Can you work these out from the model? Positions are in its coordinate system, mm. Face numbers are marked on the shaded views. Give positions to 0.01 mm unless a question says otherwise; leave off trailing zeros. Order: outer loops, then holes, each group sorted by start corner. A loop starts at its lowest first (then second) coordinate and runs counter-clockwise, first axis right, second up. Notation, with made-up numbers: (19, 57.5) - (34, 57.5) arc R27 ccw to (34, 90.5) - close; hole circle Ø5 at (88.5, 8.25). An arc over 180 degrees is marked (long way). Answer as CSV lines item,"result".
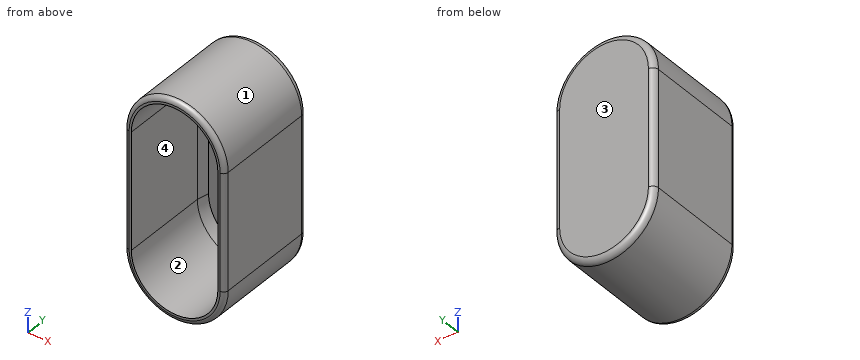
```python
from build123d import *

# Parameters (mm, degrees)
F1_DEPTH  = 15
F5_DEPTH  = 2
F10_DEPTH = 1.5
F11_R     = 1
F12_R     = 0.8


with BuildPart() as f1:
    # F0 (on Front) → F1 (new body)
    with BuildSketch(Plane.XZ):
        with BuildLine():
            Line((8.8, 0), (8.8, 20.5))
            ThreePointArc((8.8, 20.5), (0, 29.3), (-8.8, 20.5))
            Line((-8.8, 20.5), (-8.8, 0))
            ThreePointArc((-8.8, 0), (0, -8.8), (8.8, 0))
        make_face()
        with BuildLine():
            ThreePointArc((-7.6, 20.5), (0, 28.1), (7.6, 20.5))
            Line((7.6, 20.5), (7.6, 0))
            ThreePointArc((7.6, 0), (0, -7.6), (-7.6, 0))
            Line((-7.6, 0), (-7.6, 20.5))
        make_face(mode=Mode.SUBTRACT)
    extrude(amount=F1_DEPTH)

    # F4 (on face) → F5 (join)
    with BuildSketch(Plane(origin=(0, 0, 0), x_dir=(-1, 0, 0), z_dir=(0, 1, 0))):
        with BuildLine():
            ThreePointArc((8.8, 20.5), (0, 29.3), (-8.8, 20.5))
            Line((-8.8, 20.5), (-8.8, 0))
            ThreePointArc((-8.8, 0), (0, -8.8), (8.8, 0))
            Line((8.8, 0), (8.8, 20.5))
        make_face()
    extrude(amount=F5_DEPTH)

    # F3 (on offset) → F8 section 0
    with BuildSketch(Plane(origin=(0, 2.4, 0), x_dir=(-1, 0, 0), z_dir=(0, 1, 0))):
        with BuildLine():
            ThreePointArc((7.1, 20.5), (0, 27.6), (-7.1, 20.5))
            Line((-7.1, 20.5), (-7.1, 0))
            ThreePointArc((-7.1, 0), (0, -7.1), (7.1, 0))
            Line((7.1, 0), (7.1, 20.5))
        make_face()
    # F7 (on offset) → F8 section 1
    with BuildSketch(Plane(origin=(0, 0, 0), x_dir=(-1, 0, 0), z_dir=(0, 1, 0))):
        with BuildLine():
            Line((7.6, 0), (7.6, 20.5))
            ThreePointArc((7.6, 20.5), (0, 28.1), (-7.6, 20.5))
            Line((-7.6, 20.5), (-7.6, 0))
            ThreePointArc((-7.6, 0), (0, -7.6), (7.6, 0))
        make_face()
    loft(mode=Mode.SUBTRACT)

    # F9 (on face) → F10 (join)
    with BuildSketch(Plane(origin=(0, 2, 0), x_dir=(-1, 0, 0), z_dir=(0, 1, 0))):
        with BuildLine():
            ThreePointArc((8.8, 20.5), (0, 29.3), (-8.8, 20.5))
            Line((-8.8, 20.5), (-8.8, 0))
            ThreePointArc((-8.8, 0), (0, -8.8), (8.8, 0))
            Line((8.8, 0), (8.8, 20.5))
        make_face()
    extrude(amount=F10_DEPTH)

    # F11
    f11_edges = [f1.edges().sort_by_distance(p)[0] for p in [
        (0, 3.5, -8.8),
    ]]
    fillet(f11_edges, radius=F11_R)

    # F12
    f12_edges = [f1.edges().sort_by_distance(p)[0] for p in [
        (8.8, -15, 10.25),
    ]]
    fillet(f12_edges, radius=F12_R)


solid = f1.part
```
1) I want a section at D-D on y = 1.5. Write out the boundary of the cut face in (x, z) (1 decimal).
Answer block:
outline,"(-8.8, 0) arc R8.8 ccw to (8.8, 0) - (8.8, 20.5) arc R8.8 ccw to (-8.8, 20.5) - close; hole (-7.3, 0) arc R7.3 ccw to (7.3, 0) - (7.3, 20.5) arc R7.3 ccw to (-7.3, 20.5) - close"
2) I want a section at A-A on y = -10.5. Write out the boundary of the cut face in (x, z).
Answer block:
outline,"(-8.8, 0) arc R8.8 ccw to (8.8, 0) - (8.8, 20.5) arc R8.8 ccw to (-8.8, 20.5) - close; hole (-7.6, 0) arc R7.6 ccw to (7.6, 0) - (7.6, 20.5) arc R7.6 ccw to (-7.6, 20.5) - close"
3) If we mould it in two halves opening along X, with no side actions, what happens to the marked faces 1, 2, 3 and 4? For each: +X half, -X half, draft (parallel to the pull), parting line (faces both ways), or undercut.
Answer block:
face 1,"parting line"
face 2,"undercut"
face 3,"draft"
face 4,"undercut"
4) I need wall thicknesses on line 1 along X through (y, z) = (-2.75, 6); line 2 along Y through (x, z) = (-1.75, 18.5); line 3 along Z through (x, y) = (4, -7). Which ranges of each line are inside material? Lowest first, please. Write a range as [from, to].
Answer block:
line 1,"[-8.8, -7.6], [7.6, 8.8]"
line 2,"[2, 3.5]"
line 3,"[-7.84, -6.46], [26.96, 28.34]"
5) I'm going to push flat-ended pins straight in: P1, Ø3, axis at y = -6, z = 24, coming from the -X side; P2, Ø2, axis at x = 5, y = -6, coming from the -Z side; P3, Ø4, axis at x = 2.5, y = -5, coming from the -Z side. Where does each tip first touch, or does it pass through?
Answer block:
P1,"x = -8.57"
P2,"z = -7.84"
P3,"z = -8.79"
6) I want a section at C-C on z = 7. Write out the boundary of the cut face in (x, y), plus the area to 3 significant figures.
Answer block:
outline,"(-8.8, -14.2) arc R0.8 ccw to (-8, -15) - (-7.6, -15) - (-7.6, 0) - (-7.18, 2) - (7.18, 2) - (7.6, 0) - (7.6, -15) - (8, -15) arc R0.8 ccw to (8.8, -14.2) - (8.8, 2.5) arc R1 ccw to (7.8, 3.5) - (-7.8, 3.5) arc R1 ccw to (-8.8, 2.5) - close"
area,"67.3 mm2"
7) I want a section at B-B on x = 0. Write out the boundary of the cut face in (y, z), plus the area to 3 significant figures.
Answer block:
outline,"(-15, -8) arc R0.8 ccw to (-14.2, -8.8) - (2.5, -8.8) arc R1 ccw to (3.5, -7.8) - (3.5, 28.3) arc R1 ccw to (2.5, 29.3) - (-14.2, 29.3) arc R0.8 ccw to (-15, 28.5) - (-15, 28.1) - (0, 28.1) - (2, 27.68) - (2, -7.18) - (0, -7.6) - (-15, -7.6) - close"
area,"98.1 mm2"
